from build123d import *

# Parameters (mm, degrees)
EXTRUDE_1_DEPTH          = 26
SKETCH_2_R               = 3.5
SKETCH_2_R_2             = 1.6
SKETCH_2_R_3             = 2
CUT_EXTRUDE_2_DEPTH      = 155.518607294
CUT_EXTRUDE_5_DEPTH      = 155.518607294
SKETCH_5_R               = 10.5
CUT_EXTRUDE_6_DEPTH      = 1.6
CUT_EXTRUDE_START        = -1.6
SKETCH_6_R               = 10.5
CUT_EXTRUDE_7_DEPTH      = 1.6
SKETCH_7_R               = 10.5
CUT_EXTRUDE_8_DEPTH      = 1.6
SKETCH_8_R               = 10.5
CUT_EXTRUDE_9_DEPTH      = 1.6
CUT_EXTRUDE_START_2      = -26
CUT_EXTRUDE_11_OUTLINE_W = 2.5
CUT_EXTRUDE_11_OUTLINE_H = 54.794138709
CUT_EXTRUDE_11_DEPTH     = 26
SKETCH_11_W              = 55
SKETCH_11_H              = 30.411722582
CUT_EXTRUDE_12_DEPTH     = 155.518607294
EXTRUDE_2_DEPTH          = 26


# Read off the part's stored shape, not the designer's step: the extrude step
with BuildPart() as part:
    # Sketch 1 → Extrude 1 (new body)
    with BuildSketch(Plane(origin=(0, 0, 0), x_dir=(1, 0, 0), z_dir=(0, 1, 0))):
        with BuildLine():
            Line((0, 0), (0, 140))
            Line((0, 140), (5, 140))
            Line((5, 140), (5, 85))
            ThreePointArc((5, 85), (7.928932188, 77.928932188), (15, 75))
            Line((15, 75), (45, 75))
            ThreePointArc((45, 75), (52.071067812, 77.928932188), (55, 85))
            Line((55, 85), (55, 140))
            Line((55, 140), (60, 140))
            Line((60, 140), (60, 0))
            Line((60, 0), (55, 0))
            Line((55, 0), (55, 55))
            ThreePointArc((55, 55), (52.071067812, 62.071067812), (45, 65))
            Line((45, 65), (15, 65))
            ThreePointArc((15, 65), (7.928932188, 62.071067812), (5, 55))
            Line((5, 55), (5, 0))
            Line((5, 0), (0, 0))
        make_face()
    extrude(amount=EXTRUDE_1_DEPTH)

    # Sketch 2 → Cut-Extrude 2 (cut, through all)
    with BuildSketch(Plane(origin=(60, 0, 0), x_dir=(0, 0, -1), z_dir=(1, 0, 0))):
        with Locations((128, 13)):
            Circle(SKETCH_2_R)
        with Locations((123, 18)):
            Circle(SKETCH_2_R_2)
        with Locations((133, 18)):
            Circle(SKETCH_2_R_2)
        with Locations((133, 8)):
            Circle(SKETCH_2_R_2)
        with Locations((123, 8)):
            Circle(SKETCH_2_R_2)
        with Locations((12, 13)):
            Circle(SKETCH_2_R)
        with Locations((7, 18)):
            Circle(SKETCH_2_R_2)
        with Locations((7, 8)):
            Circle(SKETCH_2_R_2)
        with Locations((17, 8)):
            Circle(SKETCH_2_R_2)
        with Locations((17, 18)):
            Circle(SKETCH_2_R_2)
        with Locations((28, 13)):
            Circle(SKETCH_2_R_3)
        with Locations((44, 13)):
            Circle(SKETCH_2_R_3)
        with Locations(Location((96, 13, 0), (0, 0, 180))):
            Circle(SKETCH_2_R_3)
        with Locations(Location((112, 13, 0), (0, 0, 180))):
            Circle(SKETCH_2_R_3)
    extrude(amount=-CUT_EXTRUDE_2_DEPTH, mode=Mode.SUBTRACT)

    # Sketch 3 → Cut-Extrude 5 (cut, through all)
    with BuildSketch(Plane.ZY):
        with BuildLine():
            Line((-127, 26), (-140, 26))
            Line((-140, 26), (-140, 13))
            ThreePointArc((-140, 13), (-136.192388155, 22.192388155), (-127, 26))
        make_face()
        with BuildLine():
            ThreePointArc((-127, 0), (-136.192388155, 3.807611845), (-140, 13))
            Line((-140, 13), (-140, 0))
            Line((-140, 0), (-127, 0))
        make_face()
        with BuildLine():
            ThreePointArc((0, 13), (-3.807611845, 3.807611845), (-13, 0))
            Line((-13, 0), (0, 0))
            Line((0, 0), (0, 13))
        make_face()
        with BuildLine():
            Line((0, 26), (-13, 26))
            ThreePointArc((-13, 26), (-3.807611845, 22.192388155), (0, 13))
            Line((0, 13), (0, 26))
        make_face()
    extrude(amount=-CUT_EXTRUDE_5_DEPTH, mode=Mode.SUBTRACT)

    # Sketch 5 → Cut-Extrude 6 (cut)
    with BuildSketch(Plane.ZY.offset(-55)):
        with Locations((-128, 13)):
            Circle(SKETCH_5_R)
    extrude(amount=-CUT_EXTRUDE_6_DEPTH, mode=Mode.SUBTRACT)

    # Sketch 6 → Cut-Extrude 7 (cut)
    with BuildSketch(Plane(origin=(5, 0, 0), x_dir=(0, 0, -1), z_dir=(1, 0, 0)).offset(CUT_EXTRUDE_START)):
        with Locations(Location((128, 13, 0), (0, 0, 180))):
            Circle(SKETCH_6_R)
    extrude(amount=CUT_EXTRUDE_7_DEPTH, mode=Mode.SUBTRACT)

    # Sketch 7 → Cut-Extrude 8 (cut)
    with BuildSketch(Plane.ZY.offset(-55)):
        with Locations((-12, 13)):
            Circle(SKETCH_7_R)
    extrude(amount=-CUT_EXTRUDE_8_DEPTH, mode=Mode.SUBTRACT)

    # Sketch 8 → Cut-Extrude 9 (cut)
    with BuildSketch(Plane(origin=(5, 0, 0), x_dir=(0, 0, -1), z_dir=(1, 0, 0)).offset(CUT_EXTRUDE_START)):
        with Locations(Location((12, 13, 0), (0, 0, 180))):
            Circle(SKETCH_8_R)
    extrude(amount=CUT_EXTRUDE_9_DEPTH, mode=Mode.SUBTRACT)

    # Cut-Extrude 11 outline → Cut-Extrude 11 (cut)
    with BuildSketch(Plane(origin=(0, 26, 0), x_dir=(1, 0, 0), z_dir=(0, 1, 0)).offset(CUT_EXTRUDE_START_2)):
        with Locations((3.75, 27.397069355)):
            Rectangle(CUT_EXTRUDE_11_OUTLINE_W, CUT_EXTRUDE_11_OUTLINE_H)
        with Locations((56.25, 27.397069355)):
            Rectangle(CUT_EXTRUDE_11_OUTLINE_W, CUT_EXTRUDE_11_OUTLINE_H)
        with Locations((3.75, 112.602930646)):
            Rectangle(CUT_EXTRUDE_11_OUTLINE_W, CUT_EXTRUDE_11_OUTLINE_H)
        with Locations((56.25, 112.602930646)):
            Rectangle(CUT_EXTRUDE_11_OUTLINE_W, CUT_EXTRUDE_11_OUTLINE_H)
    extrude(amount=CUT_EXTRUDE_11_DEPTH, mode=Mode.SUBTRACT)

    # Sketch 11 → Cut-Extrude 12 (cut, through all)
    with BuildSketch(Plane(origin=(0, 26, 0), x_dir=(1, 0, 0), z_dir=(0, 1, 0))):
        with Locations((30, 70)):
            Rectangle(SKETCH_11_W, SKETCH_11_H)
    extrude(amount=-CUT_EXTRUDE_12_DEPTH, mode=Mode.SUBTRACT)


with BuildPart() as cut_extrude_12_piece_1:
    # of the separate pieces the step leaves, piece 1, a body of its own (cut_extrude_12_pieces)
    add(part.part.solids().sort_by_distance((60, 0, -127))[0])



with BuildPart() as cut_extrude_12_piece_2:
    # of the separate pieces the step leaves, piece 2, a body of its own (cut_extrude_12_pieces)
    add(part.part.solids().sort_by_distance((0, 26, -127))[0])


with BuildPart() as cut_extrude_12_piece_1_1:
    add(cut_extrude_12_piece_1.part)

    add(cut_extrude_12_piece_2.part)  # Extrude 2 merges Cut-Extrude 12 piece 2
    # Sketch 12 → Extrude 2 (add)
    with BuildSketch(Plane(origin=(0, 26, 0), x_dir=(1, 0, 0), z_dir=(0, 1, 0))):
        with BuildLine():
            Line((2.5, 85), (2.5, 75))
            Line((2.5, 75), (12.5, 75))
            ThreePointArc((12.5, 75), (5.428932188, 77.928932188), (2.5, 85))
        make_face()
        Polygon((2.5, 75), (2.5, 70), (2.5, 65), (12.5, 65), (47.5, 65), (57.5, 65), (57.5, 75), (47.5, 75), (12.5, 75), align=None)
        with BuildLine():
            Line((12.5, 65), (2.5, 65))
            Line((2.5, 65), (2.5, 55))
            ThreePointArc((2.5, 55), (5.428932188, 62.071067812), (12.5, 65))
        make_face()
        with BuildLine():
            Line((57.5, 65), (47.5, 65))
            ThreePointArc((47.5, 65), (54.571067812, 62.071067812), (57.5, 55))
            Line((57.5, 55), (57.5, 65))
        make_face()
        with BuildLine():
            ThreePointArc((57.5, 85), (54.571067812, 77.928932188), (47.5, 75))
            Line((47.5, 75), (57.5, 75))
            Line((57.5, 75), (57.5, 85))
        make_face()
    extrude(amount=-EXTRUDE_2_DEPTH)


solid = cut_extrude_12_piece_1_1.part
Geometry: final body of the model. Coordinates: model frame, mm. A direction names the side the tool comes from. Round coordinates to 2 decimals unless told otherwise and drop trailing zeros. Loops run counter-clockwise (first coordinate to the right, second up) from the corner with the lowest first, then second, coordinate; pieces in that order, holes last. Notation, with made-up numbers: M -31,-34.5 L 26,-34.5 A29 cw 26,-6.5 Z; hole C -20.75,65 d7. An arc over 180 degrees is marked long. One line per question, with ' | ' between items.
(1) Cut plane A-A on z = -108. Return the cut outline in (x, y), plus the area to 3 significant figures.
Check result:
outline: M 0,0 L 2.5,0 L 2.5,26 L 0,26 Z; M 57.5,0 L 60,0 L 60,26 L 57.5,26 Z | area: 130 mm2
(2) Pull-direction query (Y, two-part tool) for faces 4 (the flat face through (30, 26, -70)), 5 (the cylindrical face through (1.267, 19.586, -6.792)), 6 (the flat face through (2.5, 16, -112)); classes: +Y half, -Y half, draft (parallel to the pull), parting line (faces both ways), or undercut.
Check result:
face 4: +Y half | face 5: undercut | face 6: draft
(3) Material intervals for line 1 along Y through (x, z) = (0.7, -17); line 2 along X through (y, z) = (23.5, -114); line 3 along Y through (x, z) = (0.5, -28), sorted ascending. Write a range as from..to.
Check result:
line 1: y = 0..6.4, 9.6..16.4, 19.6..26 | line 2: x = 0..2.5, 57.5..60 | line 3: y = 0..11, 15..26
(4) Access query for faces 1 (the cylindrical face through (5.35, 13.18, -61.99)), 2 (the cylindrical face through (58.77, 14.05, -131.34)), 3 (the cylindrical face through (54.65, 13.18, -78.01)). Directions: +Z, -Z, +X, -X, +Y, -Y. A direction counts if a zero-diameter tool reaches every point of the face in a straight line with its end or side. Return the directions, or none.
Check result:
face 1: +Z, +Y, -Y | face 2: +X, -X | face 3: -Z, +Y, -Y
(5) Cut plane B-B on z = -7. Return the cut outline in (x, y).
Check result:
outline: M 0,1.47 L 2.5,1.47 L 2.5,6.4 L 0,6.4 Z; M 0,9.6 L 2.5,9.6 L 2.5,16.4 L 0,16.4 Z; M 0,19.6 L 2.5,19.6 L 2.5,24.53 L 0,24.53 Z; M 57.5,1.47 L 60,1.47 L 60,6.4 L 57.5,6.4 Z; M 57.5,9.6 L 60,9.6 L 60,16.4 L 57.5,16.4 Z; M 57.5,19.6 L 60,19.6 L 60,24.53 L 57.5,24.53 Z
(6) Contact query for flat-ended pins moving along their axis: P1, Ø3.5, axis at y = 13, z = -44, coming from the -X side; P2, Ø1.5, axis at x = 21.5, y = 18, coming from the -Z side; P3, Ø3, axis at x = 15.5, y = 21.5, coming from the +Z side. Output: stop coordinate, or through.
Check result:
P1: passes through | P2: stops at z = -75 | P3: stops at z = -65
(7) Cut plane D-D on y = 3.5. Return the cut outline in (x, z).
Check result:
outline: M 0,-135.87 L 2.5,-135.87 L 2.5,-85 A10 cw 12.5,-75 L 47.5,-75 A10 cw 57.5,-85 L 57.5,-135.87 L 60,-135.87 L 60,-4.13 L 57.5,-4.13 L 57.5,-55 A10 cw 47.5,-65 L 12.5,-65 A10 cw 2.5,-55 L 2.5,-4.13 L 0,-4.13 Z
(8) Cut plane C-C on x = 28.5. Return the cut outline in (y, z), plus the area to 3 significant figures.
Check result:
outline: M 0,-75 L 26,-75 L 26,-65 L 0,-65 Z | area: 260 mm2
